```python
from build123d import *

# Parameters (mm, degrees)
F0_R      = 6.477
F0_R_2    = 3.302
F1_DEPTH  = 6.35
F3_DEPTH  = 0.79375
F4_R      = 0.79374
F5_R      = 4.76249
F7_D      = 4
F8_COUNT  = 12
F10_DEPTH = 12.701
F12_DEPTH = 4.7625
F13_R     = 0.79374


# Not quite as in the source:
# - a fillet or chamfer is up to 0.001 mm smaller than in the source, because OpenCascade refuses the exact size


with BuildPart() as f1:
    # F0 (on Top) → F1 (new body, symmetric)
    with BuildSketch(Plane.XY):
        Circle(F0_R)
        Circle(F0_R_2, mode=Mode.SUBTRACT)
    extrude(amount=F1_DEPTH, both=True)

    # F2 (on Front) → F3 (join, symmetric)
    with BuildSketch(Plane.XZ):
        Polygon((7.9375, 4.7625), (7.9375, 6.35), (4.7625, 6.35), (4.7625, -6.35), (7.9375, -6.35), (7.9375, -4.7625), (14.2875, -4.7625), (14.2875, 0), (14.2875, 4.7625), align=None)
    extrude(amount=F3_DEPTH, both=True)

    # F4 (radius 0.79375 in the source; OpenCascade refuses exactly that, so slightly less here)
    f4_edges = [f1.edges().sort_by_distance(p)[0] for p in [
        (7.9375, 0, 6.35),
        (7.9375, 0, 4.7625),
        (7.9375, 0, -6.35),
        (7.9375, 0, -4.7625),
    ]]
    fillet(f4_edges, radius=F4_R)

    # F5 (radius 4.7625 in the source; OpenCascade refuses exactly that, so slightly less here)
    f5_edges = [f1.edges().sort_by_distance(p)[0] for p in [
        (14.2875, 0, -4.7625),
        (14.2875, 0, 4.7625),
    ]]
    fillet(f5_edges, radius=F5_R)

    # F7 (through all)
    with Locations(Plane.XZ.offset(0.79375)):
        with Locations((9.525, 0)):
            Hole(F7_D / 2)

    # F8: F1 ×12 about axis
    f8_axis = Axis((0, 0, 6.35), (0, 0, 1))


with BuildPart() as f1_1:
    add(f1.part)
    for i in range(1, F8_COUNT):
        add(f1.part.rotate(f8_axis, i * 360 / F8_COUNT))

    # F9 (on face) → F10 (cut, through all)
    with BuildSketch(Plane.XY.offset(6.35)):
        with BuildLine():
            Line((3.1894870784, 0.8546204869), (6.2563015769, 1.6763709551))
            Line((6.2563015769, 1.6763709551), (15.3340724923, 4.108752341))
            ThreePointArc((15.3340724923, 4.108752341), (-15.875, 0), (15.3340724923, -4.108752341))
            Line((15.3340724923, -4.108752341), (6.2563015769, -1.6763709551))
            Line((6.2563015769, -1.6763709551), (3.1894870784, -0.8546204869))
            Line((3.1894870784, -0.8546204869), (3.1894870784, 0.8546204869))
        make_face()
    extrude(amount=-F10_DEPTH, mode=Mode.SUBTRACT)

    # F11 (on Top) → F12 (cut, symmetric)
    with BuildSketch(Plane.XY):
        with BuildLine():
            Line((3.956190703, -1.060058104), (4.7228943276, -1.265495721))
            Line((4.7228943276, -1.265495721), (5.4895979523, -1.4709333381))
            ThreePointArc((5.4895979523, -1.4709333381), (5.68325, 0), (5.4895979523, 1.4709333381))
            Line((5.4895979523, 1.4709333381), (4.7228943276, 1.265495721))
            Line((4.7228943276, 1.265495721), (3.956190703, 1.060058104))
            ThreePointArc((3.956190703, 1.060058104), (4.09575, 0), (3.956190703, -1.060058104))
        make_face()
    extrude(amount=F12_DEPTH, both=True, mode=Mode.SUBTRACT)

    # F13 (radius 0.79375 in the source; OpenCascade refuses exactly that, so slightly less here)
    f13_edges = [f1_1.edges().sort_by_distance(p)[0] for p in [
        (5.68325, 0, -4.7625),
        (4.09575, 0, -4.7625),
        (4.09575, 0, 4.7625),
        (5.68325, 0, 4.7625),
    ]]
    fillet(f13_edges, radius=F13_R)


solid = f1_1.part
```
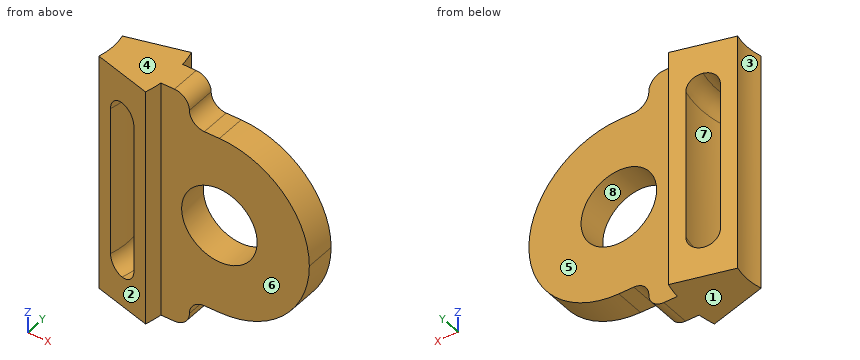
The model under review builds one solid part; all positions refer to its coordinate system, in mm. Face numbers are marked on the shaded views. A direction names the side the tool comes from. Round coordinates to 2 decimals unless told otherwise and drop trailing zeros. Loops run counter-clockwise (first coordinate to the right, second up) from the corner with the lowest first, then second, coordinate; pieces in that order, holes last.
Item 1: Clearance check with flat-ended pins moving along their axes: pin 1 Ø2.5 at (x, z) = (12, 2) entering from -Y; pin 2 Ø5 at (x, z) = (5, 4) entering from +Y; pin 3 Ø6.5 at (x, z) = (12.5, -3) entering from +Y. State where each tip first meets the part, or that it passes through.
Determined:
pin 1: stops at y = -0.79
pin 2: stops at y = 1.68
pin 3: stops at y = 0.79
Item 2: For line 1 (X direction, y = 0.6, z = 1.75); line 2 (Y direction, x = 11.75, z = 2); line 3 (X direction, y = -0.15, z = 2.5), list the stretches that pass through material, from the lowest coordinate up.
Determined:
line 1: x = 3.25 to 4.05, 5.65 to 8.56, 10.49 to 13.95
line 2: y = -0.79 to 0.79
line 3: x = 3.3 to 4.09, 5.68 to 13.58
Item 3: Take a section at D-D (x = 10.75). Write out the cut boundary in (y, z), then the cut area to 3 significant figures.
Determined:
outline: (-0.79, -4.6) - (0.79, -4.6) - (0.79, -1.58) - (-0.79, -1.58) - close; (-0.79, 1.58) - (0.79, 1.58) - (0.79, 4.6) - (-0.79, 4.6) - close
area: 9.59 mm2
Item 4: Take a section at C-C (z = 5). Write out the cut boundary in (x, y) (3 decimals), then the cut area to 3 significant figures.
Determined:
outline: (3.189, -0.855) - (6.256, -1.676) arc R6.477 ccw to (6.428, -0.794) - (8.165, -0.794) - (8.165, 0.794) - (6.428, 0.794) arc R6.477 ccw to (6.256, 1.676) - (3.189, 0.855) arc R3.302 cw to start
area: 10.8 mm2
Item 5: Mouldability with a two-part tool opening along Y and no side actions: class the marked faces 1, 2 and 3 as released by +Y, released by -Y, zero draft, split by the parting line, or undercut.
Determined:
face 1: zero draft
face 2: released by -Y
face 3: undercut
Item 6: Take a section at A-A (x = 8.5). Write out the cut boundary in (y, z).
Determined:
outline: (-0.79, -4.8) - (0.79, -4.8) - (0.79, -1.72) - (-0.79, -1.72) - close; (-0.79, 1.72) - (0.79, 1.72) - (0.79, 4.8) - (-0.79, 4.8) - close
Item 7: For the marked faces 4, 5, 6, 7 and 8, list the 3-axis set-ups (+Z, -Z, +X, -X, +Y, -Y) from which the entire face can be reached by the end or side of a thin tool; tool diameter is ignored.
Determined:
face 4: +Z, +X, -X, +Y, -Y
face 5: +Z, -Z, +X, +Y
face 6: +Z, -Z, +X, -Y
face 7: none
face 8: +Y, -Y
Item 8: Take a section at B-B (z = -2.5). Write out the cut boundary in (x, y), then the cut area to 3 significant figures.
Determined:
outline: (3.19, -0.85) - (3.96, -1.06) arc R4.1 ccw to (3.96, 1.06) - (3.19, 0.85) arc R3.3 cw to start; (5.49, -1.47) - (6.26, -1.68) arc R6.48 ccw to (6.43, -0.79) - (13.58, -0.79) - (13.58, 0.79) - (6.43, 0.79) arc R6.48 ccw to (6.26, 1.68) - (5.49, 1.47) arc R5.68 cw to start
area: 15.4 mm2
